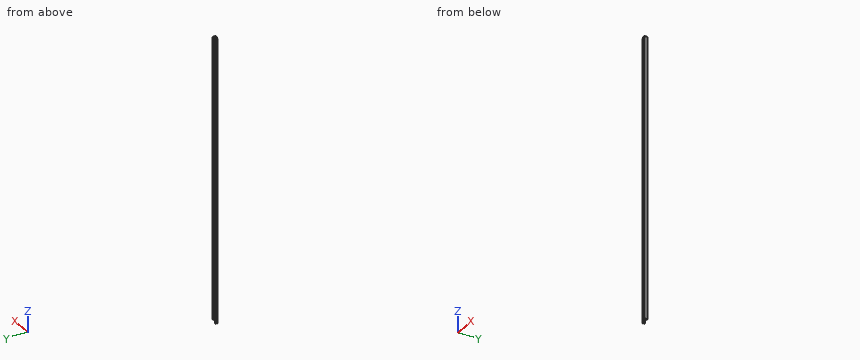
```python
from build123d import *

# Parameters (mm, degrees)
BOSS_EXTRUDE1_DEPTH = 2500
CUT_EXTRUDE2_DEPTH  = 25.4


with BuildPart() as part:
    # Sketch1 → Boss-Extrude1 (new body)
    with BuildSketch(Plane(origin=(0, 0, -3683), x_dir=(-1, 0, 0), z_dir=(0, 0, -1))):
        with BuildLine():
            Line((25.4, -5.969), (25.4, -4.826))
            ThreePointArc((25.4, -4.826), (25.176815367, -4.287184633), (24.638, -4.064))
            Line((24.638, -4.064), (23.0632, -4.064))
            ThreePointArc((23.0632, -4.064), (22.793792316, -4.175592316), (22.6822, -4.445))
            ThreePointArc((22.6822, -4.445), (22.570607684, -4.714407684), (22.3012, -4.826))
            Line((22.3012, -4.826), (13.081, -4.826))
            ThreePointArc((13.081, -4.826), (12.811592316, -4.714407684), (12.7, -4.445))
            Line((12.7, -4.445), (12.7, 4.445))
            ThreePointArc((12.7, 4.445), (12.811592316, 4.714407684), (13.081, 4.826))
            Line((13.081, 4.826), (22.3012, 4.826))
            ThreePointArc((22.3012, 4.826), (22.570607684, 4.714407684), (22.6822, 4.445))
            ThreePointArc((22.6822, 4.445), (22.793792316, 4.175592316), (23.0632, 4.064))
            Line((23.0632, 4.064), (24.638, 4.064))
            ThreePointArc((24.638, 4.064), (25.176815367, 4.287184633), (25.4, 4.826))
            Line((25.4, 4.826), (25.4, 5.969))
            ThreePointArc((25.4, 5.969), (25.288407684, 6.238407684), (25.019, 6.35))
            Line((25.019, 6.35), (13.081, 6.35))
            ThreePointArc((13.081, 6.35), (12.811592316, 6.461592316), (12.7, 6.731))
            Line((12.7, 6.731), (12.7, 10.5918))
            ThreePointArc((12.7, 10.5918), (12.082522516, 12.082522516), (10.5918, 12.7))
            Line((10.5918, 12.7), (-10.5918, 12.7))
            ThreePointArc((-10.5918, 12.7), (-12.082522516, 12.082522516), (-12.7, 10.5918))
            Line((-12.7, 10.5918), (-12.7, -10.5918))
            ThreePointArc((-12.7, -10.5918), (-12.082522516, -12.082522516), (-10.5918, -12.7))
            Line((-10.5918, -12.7), (10.5918, -12.7))
            ThreePointArc((10.5918, -12.7), (12.082522516, -12.082522516), (12.7, -10.5918))
            Line((12.7, -10.5918), (12.7, -6.731))
            ThreePointArc((12.7, -6.731), (12.811592316, -6.461592316), (13.081, -6.35))
            Line((13.081, -6.35), (25.019, -6.35))
            ThreePointArc((25.019, -6.35), (25.288407684, -6.238407684), (25.4, -5.969))
        make_face()
        with BuildLine():
            Line((11.176, 9.652), (11.176, -9.652))
            ThreePointArc((11.176, -9.652), (10.729630735, -10.729630735), (9.652, -11.176))
            Line((9.652, -11.176), (-9.652, -11.176))
            ThreePointArc((-9.652, -11.176), (-10.729630735, -10.729630735), (-11.176, -9.652))
            Line((-11.176, -9.652), (-11.176, 9.652))
            ThreePointArc((-11.176, 9.652), (-10.729630735, 10.729630735), (-9.652, 11.176))
            Line((-9.652, 11.176), (9.652, 11.176))
            ThreePointArc((9.652, 11.176), (10.729630735, 10.729630735), (11.176, 9.652))
        make_face(mode=Mode.SUBTRACT)
    extrude(amount=-BOSS_EXTRUDE1_DEPTH)

    # Sketch2 → Cut-Extrude2 (cut)
    with BuildSketch(Plane(origin=(0, 0, -3683), x_dir=(-1, 0, 0), z_dir=(0, 0, -1))):
        with BuildLine():
            Line((12.758304506, -12.7), (12.758304506, 12.7))
            Line((12.758304506, 12.7), (10.5918, 12.7))
            Line((10.5918, 12.7), (-10.5918, 12.7))
            ThreePointArc((-10.5918, 12.7), (-12.082522516, 12.082522516), (-12.7, 10.5918))
            Line((-12.7, 10.5918), (-12.7, -12.909808873))
            Line((-12.7, -12.909808873), (-10.5918, -12.7))
            Line((-10.5918, -12.7), (12.758304506, -12.7))
        make_face()
    extrude(amount=-CUT_EXTRUDE2_DEPTH, mode=Mode.SUBTRACT)


solid = part.part
```
Can you work these out from the model? Positions are in its coordinate system, mm. Coordinates: 2 decimals unless noted, no trailing zeros. Loops run counter-clockwise (first coordinate to the right, second up) from the corner with the lowest first, then second, coordinate; pieces in that order, holes last. Notation, with made-up numbers: (-12.5, 75) - (-8.5, 75) arc R15 cw to (-8.5, 97) - close; hole circle Ø10 at (-7.5, 1). An arc over 180 degrees is marked (long way). Answer as CSV lines item,"result". Start each with the question number.
1) Suppose I cut it at A-A (x = -2.5). Please give me the cut outline in (y, z), plus the area to 3 significant figures.
2) For pin 1 (8 mm diameter, centred on y = -8.5, z = -2030.5, fed in from -X); pin 2 (6 mm diameter, centred on x = -18.5, z = -2555.5, fed in from -Y); pin 3 (3.5 mm diameter, centred on x = -19, z = -2721, fed in from +Y); pin 4 (0.6 mm diameter, centred on y = 5.5, z = -3675, fed in from +X), each with a flat end and sliding along its axis, tell me the tip position at first contact or that it passes through.
3) I need wall thicknesses on line 1 (Y direction, x = -1.5, z = -3503); line 2 (Y direction, x = -22, z = -2418.5). Which ranges of each line are inside material? Lowest first, please. Write a range as from..to.
Check result:
1,outline,"(-12.7, -3657.6) - (-11.18, -3657.6) - (-11.18, -1183) - (-12.7, -1183) - close; (11.18, -3657.6) - (12.7, -3657.6) - (12.7, -1183) - (11.18, -1183) - close"
1,area,"7,540 mm²"
2,pin 1,"stops at x = -25.4"
2,pin 2,"stops at y = -6.35"
2,pin 3,"stops at y = 6.35"
2,pin 4,"stops at x = -12.76"
3,line 1,"y = -12.7..-11.18, 11.18..12.7"
3,line 2,"y = -6.35..-4.83, 4.83..6.35"
